Source: CAD feature listing. Evaluate the final solid. Frame: model axes, mm. Give positions to 0.01 mm unless a question says otherwise; leave off trailing zeros. Write each loop counter-clockwise with the first axis right and the second up, starting at its lowest first coordinate (ties: lowest second). Pieces come first, ordered by that corner, then holes. Notation, with made-up numbers: M -20,63.5 L -7,63.5 A30 cw -7,86.5 Z; hole C 26.5,4 d8. An arc over 180 degrees is marked long. Return JSON: item names as keys, results as strings.
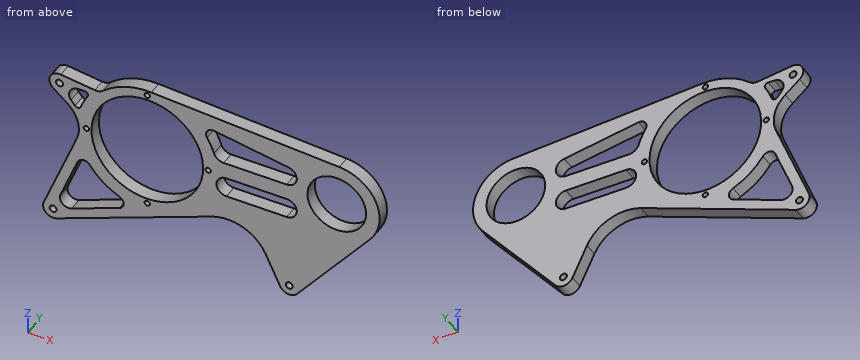
```python
from build123d import *

# Parameters (mm, degrees)
SKETCH1_R             = 52.3875
SKETCH1_R_2           = 27.49999999
BOSS_EXTRUDE1_DEPTH   = 12.7
M6_CLEARANCE_HOLE1_D  = 6.6
F_5_0MM_DOWEL_HOLE1_D = 5
CIRPATTERN1_COUNT     = 4
CUT_EXTRUDE1_DEPTH    = 285.033029848
CUT_EXTRUDE2_DEPTH    = 285.033029848


with BuildPart() as part:
    # Sketch1 → Boss-Extrude1 (new body)
    with BuildSketch(Plane(origin=(0, 0, 0), x_dir=(1, 0, 0), z_dir=(0, 1, 0))):
        with BuildLine():
            Line((-207.974881785, -9.956762437), (-62.780706514, -68.14502812))
            ThreePointArc((-62.780706514, -68.14502812), (-33.518744337, -68.231765471), (-12.176603989, -48.212200061))
            Line((-12.176603989, -48.212200061), (1.412558245, -19.284326264))
            ThreePointArc((1.412558245, -19.284326264), (8.882880061, -13.878975143), (17.431697461, -17.334586496))
            Line((17.431697461, -17.334586496), (85.833023855, -101.678807679))
            ThreePointArc((85.833023855, -101.678807679), (91.405865058, -143.189636001), (57.036931176, -167.126674473))
            Line((57.036931176, -167.126674473), (-119.452254317, -177.801047868))
            ThreePointArc((-119.452254317, -177.801047868), (-143.500663307, -174.487669009), (-164.426538493, -162.182702446))
            ThreePointArc((-164.426538493, -162.182702446), (-168.164823601, -160.06920649), (-172.443362527, -159.700770109))
            Line((-172.443362527, -159.700770109), (-204.355245166, -163.82191268))
            ThreePointArc((-204.355245166, -163.82191268), (-214.295764489, -158.206433226), (-211.707233022, -147.086764223))
            Line((-211.707233022, -147.086764223), (-198.151371623, -135.681934472))
            ThreePointArc((-198.151371623, -135.681934472), (-188.283833694, -119.954004575), (-189.430137427, -101.422354045))
            Line((-189.430137427, -101.422354045), (-220.388836369, -22.267635732))
            ThreePointArc((-220.388836369, -22.267635732), (-218.225236723, -12.034965467), (-207.974881785, -9.956762437))
        make_face()
        with Locations(Location((-123.19, -116.001477372, 0), (0, 0, 270))):
            Circle(SKETCH1_R, mode=Mode.SUBTRACT)
        with Locations(Location((54.61, -127, 0), (0, 0, 270))):
            Circle(SKETCH1_R_2, mode=Mode.SUBTRACT)
    extrude(amount=BOSS_EXTRUDE1_DEPTH)

    # M6 Clearance Hole1 (through all)
    with Locations(Plane(origin=(0, 0, 0), x_dir=(-1, 0, 0), z_dir=(0, -1, 0))):
        with Locations((-10.033704867, -23.334197365), (211.518182886, -18.798178744), (205.575185514, -154.375359311)):
            Hole(M6_CLEARANCE_HOLE1_D / 2)

    # Ø5.0mm Dowel Hole1 (through all)
    with Locations(Plane(origin=(0, 0, 0), x_dir=(-1, 0, 0), z_dir=(0, -1, 0))):
        with Locations((123.19, -173.151477372)):
            f_5_0mm_dowel_hole1 = Hole(F_5_0MM_DOWEL_HOLE1_D / 2)

    # CirPattern1: Ø5.0mm Dowel Hole1 ×4 about axis
    cirpattern1_axis = Axis((-123.19, 0, 116.001477372), (0, 1, 0))
    for i in range(1, CIRPATTERN1_COUNT):
        add(f_5_0mm_dowel_hole1.rotate(cirpattern1_axis, i * 360 / CIRPATTERN1_COUNT), mode=Mode.SUBTRACT)

    # Sketch6 → Cut-Extrude1 (cut, through all)
    with BuildSketch(Plane.XZ):
        with BuildLine():
            ThreePointArc((-188.626913597, 77.326218823), (-183.343464985, 81.400582198), (-177.265672517, 78.648182362))
            ThreePointArc((-177.265672517, 78.648182362), (-164.864290964, 65.181201114), (-149.229324423, 55.657458697))
            ThreePointArc((-149.229324423, 55.657458697), (-145.319075006, 49.625624375), (-149.386073966, 43.698348841))
            Line((-149.386073966, 43.698348841), (-194.042740287, 25.801666969))
            ThreePointArc((-194.042740287, 25.801666969), (-202.810079512, 27.579196728), (-204.660650751, 36.331409888))
            Line((-204.660650751, 36.331409888), (-188.626913597, 77.326218823))
        make_face()
        with BuildLine():
            ThreePointArc((-194.692687992, 140.689511725), (-195.773357295, 149.809803058), (-188.096484537, 154.850952212))
            Line((-188.096484537, 154.850952212), (-182.142551509, 155.01295786))
            ThreePointArc((-182.142551509, 155.01295786), (-179.298484939, 153.425933155), (-179.332786017, 150.169219243))
            ThreePointArc((-179.332786017, 150.169219243), (-182.766707481, 143.751485155), (-185.46990532, 136.993390091))
            ThreePointArc((-185.46990532, 136.993390091), (-187.940827525, 134.871620657), (-190.985681304, 136.027573744))
            Line((-190.985681304, 136.027573744), (-194.692687992, 140.689511725))
        make_face()
    extrude(amount=-CUT_EXTRUDE1_DEPTH, mode=Mode.SUBTRACT)

    # Sketch7 → Cut-Extrude2 (cut, through all)
    with BuildSketch(Plane.XZ):
        with BuildLine():
            Line((-48.815667356, 114.096477372), (7.572332644, 114.096477372))
            ThreePointArc((7.572332644, 114.096477372), (17.097332644, 104.571477372), (7.572332644, 95.046477372))
            Line((7.572332644, 95.046477372), (-48.815667356, 95.046477372))
            ThreePointArc((-48.815667356, 95.046477372), (-58.340667356, 104.571477372), (-48.815667356, 114.096477372))
        make_face()
        with BuildLine():
            Line((-60.480063265, 159.980626251), (9.143311078, 148.338049571))
            ThreePointArc((9.143311078, 148.338049571), (17.064665217, 138.155302762), (7.572332644, 129.418495204))
            Line((7.572332644, 129.418495204), (-51.525154545, 129.418495204))
            ThreePointArc((-51.525154545, 129.418495204), (-57.140513894, 131.249772802), (-60.59665397, 136.039442314))
            ThreePointArc((-60.59665397, 136.039442314), (-63.415414116, 143.322639291), (-67.078188304, 150.220062883))
            ThreePointArc((-67.078188304, 150.220062883), (-66.914295931, 157.219714512), (-60.480063265, 159.980626251))
        make_face()
    extrude(amount=-CUT_EXTRUDE2_DEPTH, mode=Mode.SUBTRACT)


solid = part.part
```
1) Cut plane B-B, the plane z = 52. Return the cut outline in (x, y).
Numbers:
{"outline": "M -208.76,0 L -198.53,0 L -198.53,12.7 L -208.76,12.7 Z; M -145.74,0 L -103.07,0 L -103.07,12.7 L -145.74,12.7 Z; M -14.21,0 L 45.54,0 L 45.54,12.7 L -14.21,12.7 Z"}
2) Cut plane C-C, the plane y = 3.5. Give the number of separate pieces and of enclosed holes in the cut face, then the cut area to 3 significant figures.
Numbers:
{"separate pieces": "1", "enclosed holes": "13", "area": "19,300 mm²"}
3) Contact query for flat-ended pins moving along their axis: pin 1 Ø4 at (x, z) = (-211.52, 18.8) entering from -Y; pin 2 Ø6 at (x, y) = (20.5, 6.5) entering from -Z; pin 3 Ø5 at (y, z) = (8, 102) entering from +X; pin 4 Ø1.5 at (x, y) = (-114.5, 2) entering from -Z. Output: stop coordinate, or through.
Numbers:
{"pin 1": "passes through", "pin 2": "stops at z = 17.42", "pin 3": "stops at x = 87.92", "pin 4": "stops at z = 47.12"}
4) Cut plane D-D, the plane x = -87.5. Return the cut outline in (y, z).
Numbers:
{"outline": "M 0,58.24 L 12.7,58.24 L 12.7,77.65 L 0,77.65 Z; M 0,154.35 L 12.7,154.35 L 12.7,175.87 L 0,175.87 Z"}
5) Cut plane A-A, the plane x = 46. Return the cut outline in (y, z).
Numbers:
{"outline": "M 0,52.56 L 12.7,52.56 L 12.7,100.88 L 0,100.88 Z; M 0,153.12 L 12.7,153.12 L 12.7,167.79 L 0,167.79 Z"}
6) Line query: line 1 (X direction, y = 7.25, z = 96.5); line 2 (X direction, y = 3, z = 102); line 3 (X direction, y = 10.75, z = 71.5). Output: solid intervals per line, ascending. Write a range as [from, to].
Numbers:
{"line 1": "x = [-191.36, -171.81], [-74.57, -53.87], [12.63, 81.63]", "line 2": "x = [-189.21, -173.67], [-72.71, -57.99], [16.74, 43.15], [66.07, 86.09]", "line 3": "x = [-201.13, -190.91], [-171.55, -150.83], [-95.55, 61.36]"}
